Verification items for the finished model (mm, model axes). A direction names the side the tool comes from. Give positions to 0.01 mm unless a question says otherwise; leave off trailing zeros. Order: outer loops, then holes, each group sorted by start corner. A loop starts at its lowest first (then second) coordinate and runs counter-clockwise, first axis right, second up. Notation, with made-up numbers: (3, 34.5) - (46, 34.5) arc R9 ccw to (46, 43.5) - close; hole circle Ø5 at (-13.5, -33.5). An arc over 180 degrees is marked (long way). Answer as a JSON object with one key per item and string values. Group by question number.
(1) Depth check by flat-ended pin: pin 1 Ø0.6 at (y, z) = (2, 0) entering from -X; pin 2 Ø1 at (x, y) = (14.5, 1.5) entering from -Z. Enter the tip coordinate at first touch or a pass-through.
(2) Section check A-A (x = -21). Record the boundary of the cut face in (y, z) (3 decimals).
(3) Access from +Z, -Z, +X, -X, +Y, -Y to the whole of each face (thin tool, end or side, straight path). Record for faces 1 (the face through (-21, 2, 0.541)), 2 (the face through (-32.647, 1.565, -0.406)), 3 (the face through (-5, 2, -4.372)).
(4) Section check D-D (x = 8). Record the boundary of the cut face in (y, z) (3 decimals).
(5) Section check C-C (z = 1.5). Record the boundary of the cut face in (x, y) (3 decimals).
(6) Section check B-B (y = 2.05). Record the boundary of the cut face in (x, z).
(7) Thickness scan on line 1 (X direction, y = 0.35, z = -0.5); line 2 (X direction, y = 0.65, z = 0.5); line 3 (X direction, y = 2.5, z = 0). Record the ranges inside material, lowest first.
```python
from build123d import *

# Parameters (mm, degrees)
SKETCH1_R           = 0.8763
SKETCH1_W           = 4.871922601
SKETCH1_H           = 2.01733498
BOSS_EXTRUDE1_DEPTH = 3.175


with BuildPart() as part:
    # Sketch1 → Boss-Extrude1 (new body)
    with BuildSketch(Plane(origin=(0, 0, 0), x_dir=(1, 0, 0), z_dir=(0, 1, 0))):
        with BuildLine():
            Line((19.886382458, -3.437122558), (-28.789940164, -3.436792079))
            ThreePointArc((-28.789940164, -3.436792079), (-32.647020001, 0.491263054), (-28.742479365, 4.372144967))
            Line((-28.742479365, 4.372144967), (19.886338504, 4.372144967))
            ThreePointArc((19.886338504, 4.372144967), (28.36848968, 0.467558945), (19.886382458, -3.437122558))
        make_face()
        with Locations(Location((-28.742479365, 0.467532217, 0), (0, 0, 270))):
            Circle(SKETCH1_R, mode=Mode.SUBTRACT)
        with Locations(Location((-7.951646395, 0.467466465, 0), (0, 0, 270))):
            Circle(SKETCH1_R, mode=Mode.SUBTRACT)
        with Locations(Location((23.228702339, 0.467530016, 0), (0, 0, 270))):
            Circle(SKETCH1_R, mode=Mode.SUBTRACT)
        Polygon((-22.242501784, 1.443620076), (-22.242501784, 1.476197509), (-18.994538581, 1.476197509), (-18.994538581, 1.443620076), (-18.994538581, -0.508687146), (-18.994538581, -0.541137472), (-22.242501784, -0.541137472), (-22.242501784, -0.508687146), align=None, mode=Mode.SUBTRACT)
        with Locations((14.296879657, 0.467530017)):
            Rectangle(SKETCH1_W, SKETCH1_H, mode=Mode.SUBTRACT)
    extrude(amount=BOSS_EXTRUDE1_DEPTH)


solid = part.part
```
Solutions:
{
 "1": {"pin 1": "stops at x = -32.64", "pin 2": "stops at z = -4.37"},
 "2": {"outline": "(0, -4.372) - (3.175, -4.372) - (3.175, -1.476) - (0, -1.476) - close; (0, 0.541) - (3.175, 0.541) - (3.175, 3.437) - (0, 3.437) - close"},
 "3": {"face 1": "+Y, -Y", "face 2": "-X, +Y, -Y", "face 3": "-Z, -X, +Y, -Y"},
 "4": {"outline": "(0, -4.372) - (3.175, -4.372) - (3.175, 3.437) - (0, 3.437) - close"},
 "5": {"outline": "(-32.115, 0) - (27.977, 0) - (27.977, 3.175) - (-32.115, 3.175) - close"},
 "6": {"outline": "(-28.79, 3.44) arc R3.9 ccw to (-28.74, -4.37) - (19.89, -4.37) arc R5.14 ccw (long way) to (19.89, 3.44) - close; hole circle Ø1.75 at (-28.74, -0.47); hole (-22.24, -1.48) - (-18.99, -1.48) - (-18.99, 0.54) - (-22.24, 0.54) - close; hole circle Ø1.75 at (-7.95, -0.47); hole (11.86, -1.48) - (16.73, -1.48) - (16.73, 0.54) - (11.86, 0.54) - close; hole circle Ø1.75 at (23.23, -0.47)"},
 "7": {"line 1": "x = -32.65 to -29.62, -27.87 to -22.24, -18.99 to -8.83, -7.08 to 11.86, 16.73 to 22.35, 24.1 to 28.37", "line 2": "x = -32.53 to -22.24, -18.99 to 11.86, 16.73 to 28.28", "line 3": "x = -32.62 to -29.48, -28 to -22.24, -18.99 to -8.69, -7.21 to 11.86, 16.73 to 22.49, 23.97 to 28.35"}
}
